Work out the finished part from the listing and answer in its coordinate system (mm). A direction names the side the tool comes from. Coordinates: 2 decimals unless noted, no trailing zeros. Loops run counter-clockwise (first coordinate to the right, second up) from the corner with the lowest first, then second, coordinate; pieces in that order, holes last. Notation, with made-up numbers: (54, 77.5) - (86, 77.5) arc R21 ccw to (86, 100.5) - close; hole circle Ø9 at (54.25, -29). An arc over 180 degrees is marked (long way). Write each question's results on one line, items separated by ' | '. Start each with the question number.
1. A cutting plane is placed at B-B on x = 0. Determine the outline of the cut face in (y, z).
2. A cutting plane is placed at D-D on y = 3.5. Determine the outline of the cut face in (x, z), then the cut area to 3 significant figures.
3. Each of these flat-tipped pins is pushed along its axis until it touches: P1, Ø6, axis at y = 5.5, z = -2.5, coming from the +X side; P2, Ø1, axis at x = -8.5, y = -1, coming from the +Z side; P3, Ø2, axis at y = -0.5, z = 4.5, coming from the +X side. Where does it stop, or does it pass through?
4. Which of the six approach directions +Z, -Z, +X, -X, +Y, -Y give full straight-line access (tool end or side, diameter ignored) to faces 4 (the flat face through (0, 0, 0)), 5 (the cylindrical face through (1.802, 15.776, 5.723)), 6 (the flat face through (0, 32, 0))?
5. Find the intervals of material crossed by line 1 along X through (y, z) = (-3.5, 0); line 2 along Y through (x, z) = (8, -3.5); line 3 along X through (y, z) = (-5, -11.25), in increasing order. Write a range as [from, to].
6. A cutting plane is placed at C-C on y = -11. Determine the outline of the cut face in (x, z).
7. Determine the mould class of faces 1 (the cylindrical face through (-2.44, -7.89, 0.54)), 2 (the cylindrical face through (-13.67, -7.89, 3.03)), 3 (the flat face through (0, -16, -3)) for opening direction Z: released by +Z, released by -Z, zero draft, split by the parting line, or undercut.
8. A cutting plane is placed at A-A on z = 0. Determine the outline of the cut face in (x, y).
from build123d import *

# Parameters (mm, degrees)
SKETCH_1_R      = 6
EXTRUDE_1_DEPTH = 32
SKETCH_3_R      = 14
SKETCH_3_R_2    = 2.5
EXTRUDE_2_DEPTH = 16


with BuildPart() as part:
    # 草图1 → 凸台-拉伸1 (new body)
    with BuildSketch(Plane(origin=(0, 0, 0), x_dir=(1, 0, 0), z_dir=(0, 1, 0))):
        with Locations(Location((0, 0, 0), (0, 0, 270))):
            Circle(SKETCH_1_R)
    extrude(amount=EXTRUDE_1_DEPTH)

    # 草图3 → 凸台-拉伸2 (add)
    with BuildSketch(Plane.XZ):
        with Locations(Location((0, 0, 0), (0, 0, 270))):
            Circle(SKETCH_3_R)
        with Locations(Location((0, 0, 0), (0, 0, 270))):
            Circle(SKETCH_3_R_2, mode=Mode.SUBTRACT)
    extrude(amount=EXTRUDE_2_DEPTH)


solid = part.part
Values:
1) outline: (-16, -14) - (0, -14) - (0, -6) - (32, -6) - (32, 6) - (0, 6) - (0, 14) - (-16, 14) - (-16, 2.5) - (0, 2.5) - (0, -2.5) - (-16, -2.5) - close
2) outline: circle Ø12 at (0, 0) | area: 113 mm^2
3) P1: x = 6 | P2: z = 11.49 | P3: x = 13.56
4) face 4: -Y | face 5: +Y | face 6: +Z, -Z, +X, -X, +Y
5) line 1: [-14, -2.5], [2.5, 14] | line 2: [-16, 0] | line 3: [-8.33, 8.33]
6) outline: circle Ø28 at (0, 0); hole circle Ø5 at (0, 0)
7) face 1: undercut | face 2: split by the parting line | face 3: zero draft
8) outline: (-14, -16) - (-2.5, -16) - (-2.5, 0) - (2.5, 0) - (2.5, -16) - (14, -16) - (14, 0) - (6, 0) - (6, 32) - (-6, 32) - (-6, 0) - (-14, 0) - close
